Model file for the job. Use its own axes, mm. Face numbers are marked on the shaded views. A direction names the side the tool comes from. Round coordinates to 2 decimals unless told otherwise and drop trailing zeros. Order: outer loops, then holes, each group sorted by start corner. A loop starts at its lowest first (then second) coordinate and runs counter-clockwise, first axis right, second up. Notation, with made-up numbers: (-4.75, 20) - (54.25, 20) arc R32 ccw to (54.25, 50) - close; hole circle Ø7 at (-28, 71.25). An arc over 180 degrees is marked (long way). Answer as CSV lines item,"result". Start each with the question number.
1. Pull direction X, two halves, no side cores. Call the marked faces 4, 5, 6 and 7: released by +X, released by -X, zero draft, split by the parting line, or undercut.
2. Band-saw the part on A-A on z = -8.5. List the corners of the cut face in (x, y).
3. Band-saw the part on B-B on y = -67. List the corners of the cut face in (x, z).
4. 3-axis set-ups, long thin cutter, end or side, ignore diameter. For the marked faces 1, 2 and 3: which of +Z, -Z, +X, -X, +Y, -Y reach the whole face in a straight line?
5. Band-saw the part on C-C on x = 45. List the corners of the cut face in (y, z).
6. Pin check, flat tips, straight feed: pin 1 Ø1 at (y, z) = (-35, -26) entering from -X; pin 2 Ø4 at (x, y) = (-74.5, -17.5) entering from +Z; pin 3 Ø3 at (y, z) = (-23.5, -32.5) entering from -X. Stop position of each tip, or through.
7. Band-saw the part on D-D on z = -46. List the corners of the cut face in (x, y) (1 decimal).
8. Wall check: line 1 along X through (y, z) = (-33, -1); line 2 along Y through (x, z) = (45, -1.7); line 3 along Y through (x, z) = (-81.5, -5.5). Give the ranges that are in metal, low to high. Write a range as [from, to].
Autodesk Inventor part; units mm, degrees
ref_plane "Work Plane1" through (0, 0, -32) normal (0, 0, 1) x (1, 0, 0)
ref_plane "YZ Plane" through (0, 0, 0) normal (1, 0, 0) x (0, 1, 0)
ref_plane "XZ Plane" through (0, 0, 0) normal (0, 1, 0) x (-1, 0, 0)
sketch "Sketch1" plane through (0, 0, 0) normal (0, 0, 1) x (1, 0, 0)
  line L0 (1.6571, 0) -> (65, 0)
  arc A0 (78.6808, -77.5877) -> (65, 0) centre (65, -40) ccw
  line L1 (65, -40) -> (78.6808, -77.5877) construction
  line L2 (65, -40) -> (65, 0) construction
  arc A1 (-0.3126, -1.6535) -> (78.6808, -77.5877) centre (64.6893, -13.0878) ccw
  arc A2 (1.6571, 0) -> (-0.3126, -1.6535) centre (1.6571, -2) ccw
  line L3 (65, -3) -> (2.5022, -3)
  arc A3 (2.5022, -3) -> (77.8443, -74.699) centre (64.6893, -13.0878) ccw
  arc A4 (77.8443, -74.699) -> (65, -3) centre (65, -40) ccw
  point P0 (0, 0)
  dimension "d4" = 65
  dimension "d5" = 160
  dimension "d6" = 66
  dimension "d8" = 2
  dimension "d11" = 3
extrude "Extrusion1" add sketch "Sketch1" against normal blind 60 contours L0 A0 A1 A2 | A4 A3 L3
extrude "Extrusion2" cut sketch "Sketch1" against normal blind 2 contours A4 A3 L3
sketch "Sketch3" plane through (0, 0, -2) normal (0, 0, 1) x (1, 0, 0)
  circle A0 centre (45, -33) radius 25
  circle A1 centre (45, -33) radius 22
  point P0 (0, 0)
  dimension "d14" = 50
  dimension "d15" = 3
extrude "Extrusion3" add sketch "Sketch3" along normal blind 0.5
ref_plane "Work Plane1" through (0, 0, -32) normal (0, 0, 1) x (1, 0, 0)
sketch "Sketch4" plane through (0, 0, -32) normal (0, 0, 1) x (1, 0, 0)
  arc A0 (-0.3126, -1.6535) -> (78.6808, -77.5877) centre (64.6893, -13.0878) ccw
  line L0 (-0.3126, -24.5221) -> (-7.8126, -24.5221)
  line L1 (-7.8126, -24.5221) -> (-7.8126, -59.5221)
  arc A1 (-7.8126, -59.5221) -> (5.3698, -42.0221) centre (-11.6048, -42.9504) ccw
  point P0 (0, 0)
  dimension "d19" = 7.5
  dimension "d20" = 35
  dimension "d21" = 17
extrude "Extrusion4" add sketch "Sketch4" along normal mid plane 40
mirror "Mirror1" about plane through (-7.8126, -24.5221, -32) normal (-1, 0, 0)
properties part number "Project eyes"
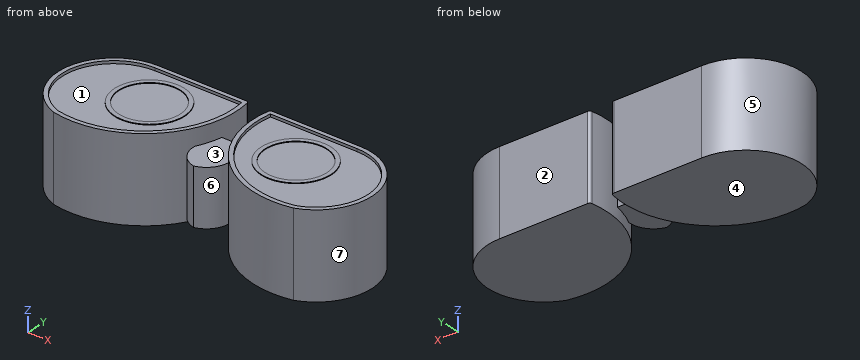
Reply:
1,face 4,"zero draft"
1,face 5,"released by -X"
1,face 6,"undercut"
1,face 7,"released by +X"
2,outline,"(-94.31, -77.59) arc R66 ccw to (-15.31, -1.65) arc R2 ccw to (-17.28, 0) - (-80.63, 0) arc R40 ccw to start; (-0.31, -1.65) arc R66 ccw to (78.68, -77.59) arc R40 ccw to (65, 0) - (1.66, 0) arc R2 ccw to start"
3,outline,"(-110.14, -60) - (-42.24, -60) - (-42.24, 0) - (-47.72, 0) - (-47.72, -2) - (-105.92, -2) - (-105.92, 0) - (-110.14, 0) - close; (26.62, -60) - (94.51, -60) - (94.51, 0) - (90.3, 0) - (90.3, -2) - (32.09, -2) - (32.09, 0) - (26.62, 0) - close"
4,face 1,"+Z"
4,face 2,"+Z, -Z, +X, -X, +Y"
4,face 3,"+Z, -Y"
5,outline,"(-76.08, -60) - (0, -60) - (0, 0) - (-3, 0) - (-3, -2) - (-8, -2) - (-8, -1.5) - (-11, -1.5) - (-11, -2) - (-55, -2) - (-55, -1.5) - (-58, -1.5) - (-58, -2) - (-72.93, -2) - (-72.93, 0) - (-76.08, 0) - close"
6,pin 1,"stops at x = -120.37"
6,pin 2,"stops at z = -1.5"
6,pin 3,"stops at x = -117.71"
7,outline,"(-94.3, -77.6) arc R66 ccw to (-21, -42) arc R17 ccw to (-7.8, -59.5) arc R17 ccw to (5.4, -42) arc R66 ccw to (78.7, -77.6) arc R40 ccw to (65, 0) - (1.7, 0) arc R2 ccw to (-0.3, -1.7) arc R66 ccw to (-0.3, -24.5) - (-15.3, -24.5) arc R66 ccw to (-15.3, -1.7) arc R2 ccw to (-17.3, 0) - (-80.6, 0) arc R40 ccw to start"
8,line 1,"x = [-120.01, -116.96], [-20.54, -17.39], [1.76, 4.92], [101.33, 104.38]"
8,line 2,"y = [-76.08, -72.93], [-58, -55], [-11, -8], [-3, 0]"
8,line 3,"y = [-79.08, -0.01]"
